```python
from build123d import *

# Parameters (mm, degrees)
PAD_DEPTH    = 20
SKETCH001_R  = 2.25
POCKET_DEPTH = 22.001


with BuildPart() as part:
    # Sketch → Pad (new body)
    with BuildSketch(Plane.XY):
        with BuildLine():
            Line((-17.5, 22), (17.5, 22))
            Line((17.5, 22), (17.5, 0))
            Line((17.5, 0), (4.05, 0))
            ThreePointArc((4.05, 0), (0, 4.05), (-4.05, 0))
            Line((-17.5, 0), (-4.05, 0))
            Line((-17.5, 0), (-17.5, 22))
        make_face()
    extrude(amount=PAD_DEPTH)

    # Sketch001 → Pocket (cut, through all)
    with BuildSketch(Plane.XZ):
        with Locations((-11, 10)):
            Circle(SKETCH001_R)
        with Locations((11, 10)):
            Circle(SKETCH001_R)
    extrude(amount=-POCKET_DEPTH, mode=Mode.SUBTRACT)


solid = part.part
```
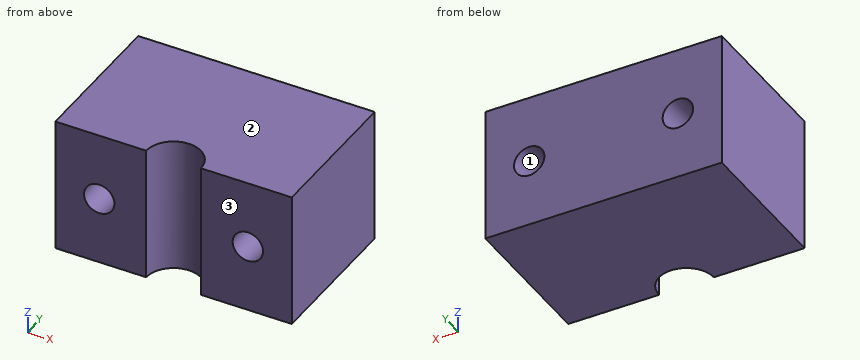
Input: part model. Units: mm. Frame: model coordinates. Face numbers are marked on the shaded views. Give positions to 0.01 mm unless a question says otherwise; leave off trailing zeros. Order: outer loops, then holes, each group sorted by start corner. A loop starts at its lowest first (then second) coordinate and runs counter-clockwise, first axis right, second up.
1. Cut plane B-B (x = -11). Return loops of the section in (y, z), and give its area (3 significant figures).
Computed:
outline: (0, 0) - (22, 0) - (22, 7.75) - (0, 7.75) - close; (0, 12.25) - (22, 12.25) - (22, 20) - (0, 20) - close
area: 341 mm2
2. Cut plane C-C (y = 18.25). Return loops of the section in (x, z).
Computed:
outline: (-17.5, 0) - (17.5, 0) - (17.5, 20) - (-17.5, 20) - close; hole circle Ø4.5 at (-11, 10); hole circle Ø4.5 at (11, 10)
3. Cut plane D-D (y = 3). Return loops of the section in (x, z), and give its area (3 significant figures).
Computed:
outline: (-17.5, 0) - (-2.72, 0) - (-2.72, 20) - (-17.5, 20) - close; (2.72, 0) - (17.5, 0) - (17.5, 20) - (2.72, 20) - close; hole circle Ø4.5 at (-11, 10); hole circle Ø4.5 at (11, 10)
area: 559 mm2
4. Cut plane A-A (z = 10). Return loops of the section in (x, y).
Computed:
outline: (-17.5, 0) - (-13.25, 0) - (-13.25, 22) - (-17.5, 22) - close; (-8.75, 0) - (-4.05, 0) arc R4.05 cw to (4.05, 0) - (8.75, 0) - (8.75, 22) - (-8.75, 22) - close; (13.25, 0) - (17.5, 0) - (17.5, 22) - (13.25, 22) - close
5. Draft query along Z for the marked faces 1, 2 and 3. Return one class per face: released by +Z, released by -Z, zero draft, split by the parting line, or undercut.
Computed:
face 1: undercut
face 2: released by +Z
face 3: zero draft
6. Line query: probe 1 along Z at (x, y) = (-11, 8); probe 2 along X at (y, z) = (16.25, 8); probe 3 along Z at (x, y) = (-12.5, 1.75). Output: solid intervals per line, ascending.
Computed:
probe 1: z = 0 to 7.75, 12.25 to 20
probe 2: x = -17.5 to -12.03, -9.97 to 9.97, 12.03 to 17.5
probe 3: z = 0 to 8.32, 11.68 to 20
7. Pin query (flat end, axial travel): pin 1 Ø7 at (x, z) = (11, 10) entering from -Y; pin 2 Ø3.5 at (x, z) = (-11, 10) entering from -Y. Return the tip coordinate at first contact, or that it passes through.
Computed:
pin 1: stops at y = 0
pin 2: passes through
